from build123d import *

# Parameters (mm, degrees)
SKETCH_1_W          = 77
SKETCH_1_H          = 61
EXTRUDE_1_DEPTH     = 2
SKETCH_2_W          = 28
SKETCH_2_H          = 11
CUT_EXTRUDE_1_DEPTH = 99.254770877
SKETCH_3_W          = 10
SKETCH_3_H          = 5
SKETCH_3_W_2        = 8
SKETCH_3_H_2        = 6.5
SKETCH_3_H_3        = 8
CUT_EXTRUDE_2_DEPTH = 99.254770877
SKETCH_4_R          = 1.35
CUT_EXTRUDE_3_DEPTH = 99.254770877


with BuildPart() as part:
    # 草图1 → 凸台-拉伸1 (new body)
    with BuildSketch(Plane.XY):
        with Locations((38.5, 30.5)):
            Rectangle(SKETCH_1_W, SKETCH_1_H)
    extrude(amount=EXTRUDE_1_DEPTH)

    # 草图2 → 切除-拉伸1 (cut, through all)
    with BuildSketch(Plane.XY):
        with Locations((53.5, 10.4)):
            Rectangle(SKETCH_2_W, SKETCH_2_H)
    extrude(amount=CUT_EXTRUDE_1_DEPTH, mode=Mode.SUBTRACT)

    # 草图3 → 切除-拉伸2 (cut, through all)
    with BuildSketch(Plane.XY):
        with Locations((19.5, 53)):
            Rectangle(SKETCH_3_W, SKETCH_3_H)
        with Locations((54.5, 53.75)):
            Rectangle(SKETCH_3_W_2, SKETCH_3_H_2)
        with Locations((66.5, 39)):
            Rectangle(SKETCH_3_W_2, SKETCH_3_H_3)
    extrude(amount=CUT_EXTRUDE_2_DEPTH, mode=Mode.SUBTRACT)

    # 草图4 → 切除-拉伸3 (cut, through all)
    with BuildSketch(Plane.XY):
        with Locations((6.5, 18)):
            Circle(SKETCH_4_R)
        with Locations((70.5, 18)):
            Circle(SKETCH_4_R)
        with Locations((6.5, 54)):
            Circle(SKETCH_4_R)
        with Locations((70.5, 54)):
            Circle(SKETCH_4_R)
    extrude(amount=CUT_EXTRUDE_3_DEPTH, mode=Mode.SUBTRACT)


solid = part.part
Geometry check sheet. Reference: the model listing, model coordinates, mm. A direction names the side the tool comes from. Coordinates: 2 decimals unless noted, no trailing zeros. Loops run counter-clockwise (first coordinate to the right, second up) from the corner with the lowest first, then second, coordinate; pieces in that order, holes last. Notation, with made-up numbers: (15, -39) - (43, -39) arc R23 ccw to (43, -25) - close; hole circle Ø7 at (-17, 23). An arc over 180 degrees is marked (long way). Use one line per item in the form item = value. Start each with the question number.
Item 1: Mould release check, pull along X, two halves, no side actions. Record for faces 1 (the face through (77, 30, 1)), 2 (the face through (38, 31, 0)), 3 (the face through (53, 4.9, 1)): +X half, -X half, draft (parallel to the pull), parting line (faces both ways), or undercut.
Item 2: Gauge pin test, flat end, axial feed: pin 1 (1 mm diameter, centred on x = 65.5, z = 1, fed in from -Y). Record the tip position at first contact, or that the pin passes through.
Item 3: Section check D-D, the plane x = 6.5. Enter the section's corners in (y, z), and give its area (3 significant figures).
Item 4: Section check A-A, the plane x = 42.5. Enter the section's corners in (y, z).
Item 5: Section check B-B, the plane y = 18. Enter the section's corners in (x, z).
Item 6: Thickness scan on probe 1 along X at (y, z) = (18, 0.75); probe 2 along X at (y, z) = (54, 1.5); probe 3 along Y at (x, z) = (6.5, 0.5). Record the ranges inside material, lowest first.
Item 7: Section check C-C, the plane z = 0.5. Give the number of separate pieces and of enclosed holes in the cut face, and give its area (3 significant figures).
Item 8: Tool access check on faces 4 (the face through (38, 61, 1)), 5 (the face through (50.5, 54, 1)). Record the directions out of +Z, -Z, +X, -X, +Y, -Y that give a thin tool (end or side, any length) a straight path to the whole face; none if there is none.
Computed:
q1.face_1 = +X half
q1.face_2 = draft
q1.face_3 = undercut
q2.pin_1 = 0
q3.outline = (0, 0) - (16.65, 0) - (16.65, 2) - (0, 2) - close; (19.35, 0) - (52.65, 0) - (52.65, 2) - (19.35, 2) - close; (55.35, 0) - (61, 0) - (61, 2) - (55.35, 2) - close
q3.area = 111 mm2
q4.outline = (0, 0) - (4.9, 0) - (4.9, 2) - (0, 2) - close; (15.9, 0) - (61, 0) - (61, 2) - (15.9, 2) - close
q5.outline = (0, 0) - (5.15, 0) - (5.15, 2) - (0, 2) - close; (7.85, 0) - (69.15, 0) - (69.15, 2) - (7.85, 2) - close; (71.85, 0) - (77, 0) - (77, 2) - (71.85, 2) - close
q6.probe_1 = 0 to 5.15, 7.85 to 69.15, 71.85 to 77
q6.probe_2 = 0 to 5.15, 7.85 to 14.5, 24.5 to 50.5, 58.5 to 69.15, 71.85 to 77
q6.probe_3 = 0 to 16.65, 19.35 to 52.65, 55.35 to 61
q7.separate_pieces = 1
q7.enclosed_holes = 8
q7.area = 4,200 mm2
q8.face_4 = +Z, -Z, +X, -X, +Y
q8.face_5 = +Z, -Z
